Verification items for the finished model (mm, model axes). Face numbers are marked on the shaded views. A direction names the side the tool comes from. Round coordinates to 2 decimals unless told otherwise and drop trailing zeros. Order: outer loops, then holes, each group sorted by start corner. A loop starts at its lowest first (then second) coordinate and runs counter-clockwise, first axis right, second up. Notation, with made-up numbers: M 4.25,58 L 53.25,58 A18 cw 53.25,78 Z; hole C 72.5,34.5 d9. An arc over 180 degrees is marked long. One line per item, written item: value. Start each with the question number.
from build123d import *

# Parameters (mm, degrees)
SKETCH1_W           = 16
SKETCH1_H           = 48
SKETCH1_R           = 2.15
SKETCH1_R_2         = 1.75
BOSS_EXTRUDE1_DEPTH = 10
SKETCH2_R           = 6
BOSS_EXTRUDE2_DEPTH = 16
CHAMFER1_SIZE       = 10


with BuildPart() as part:
    # Sketch1 → Boss-Extrude1 (new body)
    with BuildSketch(Plane(origin=(0, 0, 0), x_dir=(0, 0, -1), z_dir=(1, 0, 0))):
        with Locations((8, 24)):
            Rectangle(SKETCH1_W, SKETCH1_H)
        with Locations((8, 40)):
            Circle(SKETCH1_R, mode=Mode.SUBTRACT)
        with Locations((8, 8)):
            Circle(SKETCH1_R_2, mode=Mode.SUBTRACT)
    extrude(amount=BOSS_EXTRUDE1_DEPTH)

    # Sketch2 → Boss-Extrude2 (add, through all)
    with BuildSketch(Plane.XY):
        Polygon((10, 20), (10, 0), (0, 0), (0, -6), (30, -6), (30, 20), align=None)
        with Locations((17, 3.936401072)):
            Circle(SKETCH2_R, mode=Mode.SUBTRACT)
    extrude(amount=-BOSS_EXTRUDE2_DEPTH)

    # Chamfer1
    chamfer1_edges = [part.edges().sort_by_distance(p)[0] for p in [
        (10, 20, -8),
    ]]
    chamfer(chamfer1_edges, length=CHAMFER1_SIZE)


solid = part.part
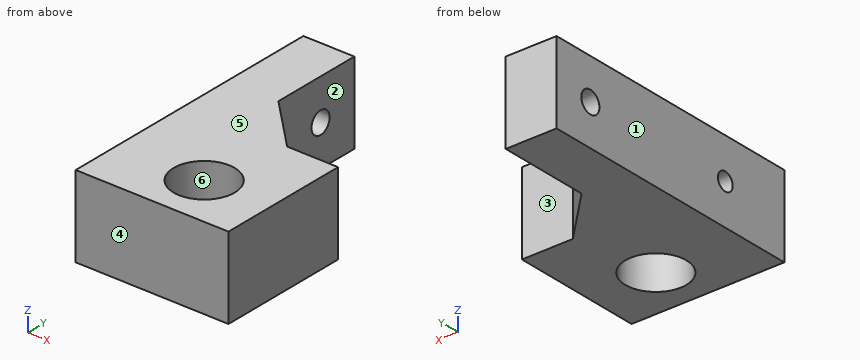
1. Scan lines: line 1 along Y through (x, z) = (2.5, -8); line 2 along Y through (x, z) = (17, -4.75); line 3 along X through (y, z) = (35, -10.5). Record each from-to range of solid material in increasing order.
2. Section check D-D (x = 5.5). Record the cut outline in (y, z), and give its area (3 significant figures).
3. Section check C-C (x = 17). Record the cut outline in (y, z), and give its area (3 significant figures).
4. Depth check by flat-ended pin: pin 1 (2 mm diameter, centred on x = 25.5, z = -7, fed in from +Y); pin 2 (8 mm diameter, centred on y = 34.5, z = -4, fed in from +X); pin 3 (6 mm diameter, centred on x = 20.5, z = -10.5, fed in from +Y). Enter the tip coordinate at first touch or a pass-through.
5. Section check B-B (z = -8). Record the cut outline in (x, y).
6. Draft check along Y on the marked faces 3, 4, 5 and 6. Enter one of: released by +Y, released by -Y, zero draft, split by the parting line, or undercut.
7. Tool access check on the marked faces 1 and 2. Record the directions out of +Z, -Z, +X, -X, +Y, -Y that give a thin tool (end or side, any length) a straight path to the whole face; none if there is none.
8. Section check A-A (y = 40). Record the cut outline in (x, z).
Geometry check:
1. line 1: y = -6 to 6.25, 9.75 to 37.85, 42.15 to 48
1. line 2: y = -6 to -2.06, 9.94 to 23
1. line 3: x = 0 to 10
2. outline: M -6,-16 L 48,-16 L 48,0 L -6,0 Z; hole C 8,-8 d3.5; hole C 40,-8 d4.3
2. area: 840 mm²
3. outline: M -6,-16 L -2.06,-16 L -2.06,0 L -6,0 Z; M 9.94,-16 L 23,-16 L 23,0 L 9.94,0 Z
3. area: 272 mm²
4. pin 1: stops at y = 20
4. pin 2: stops at x = 10
4. pin 3: stops at y = 22.5
5. outline: M 0,-6 L 30,-6 L 30,20 L 20,20 L 10,30 L 10,37.85 L 0,37.85 L 0,9.75 L 10,9.75 L 10,6.25 L 0,6.25 Z; M 0,42.15 L 10,42.15 L 10,48 L 0,48 Z; hole C 17,3.94 d12
6. face 3: released by +Y
6. face 4: released by -Y
6. face 5: zero draft
6. face 6: undercut
7. face 1: +Z, -Z, -X, +Y, -Y
7. face 2: +Z, -Z, +X, +Y
8. outline: M 0,-16 L 10,-16 L 10,-10.15 L 0,-10.15 Z; M 0,-5.85 L 10,-5.85 L 10,0 L 0,0 Z
